Geometry check sheet. Reference: the model listing, model coordinates, mm. Face numbers are marked on the shaded views. Coordinates: 2 decimals unless noted, no trailing zeros. Loops run counter-clockwise (first coordinate to the right, second up) from the corner with the lowest first, then second, coordinate; pieces in that order, holes last. Notation, with made-up numbers: (26.5, 82.25) - (61.5, 82.25) arc R22 cw to (61.5, 102.25) - close; hole circle Ø11 at (87, 64.25). An arc over 180 degrees is marked (long way). One line per item, written item: value.
from build123d import *

# Parameters (mm, degrees)
SKETCH_1_R          = 12.5
SKETCH_1_R_2        = 4
SKETCH_1_R_3        = 1.2
EXTRUDE_1_DEPTH     = 1.2
SKETCH_3_R          = 6
CUT_EXTRUDE_2_DEPTH = 0.3


with BuildPart() as part:
    # 草图1 → 凸台-拉伸1 (new body)
    with BuildSketch(Plane.XY):
        Circle(SKETCH_1_R)
        Circle(SKETCH_1_R_2, mode=Mode.SUBTRACT)
        with Locations((0, -7.5)):
            Circle(SKETCH_1_R_3, mode=Mode.SUBTRACT)
        with Locations((-6.495190528, 3.75)):
            Circle(SKETCH_1_R_3, mode=Mode.SUBTRACT)
        with Locations((6.495190528, 3.75)):
            Circle(SKETCH_1_R_3, mode=Mode.SUBTRACT)
    extrude(amount=EXTRUDE_1_DEPTH)

    # 草图3 → 切除-拉伸2 (cut)
    with BuildSketch(Plane.XY.offset(1.2)):
        Circle(SKETCH_3_R)
    extrude(amount=-CUT_EXTRUDE_2_DEPTH, mode=Mode.SUBTRACT)


solid = part.part
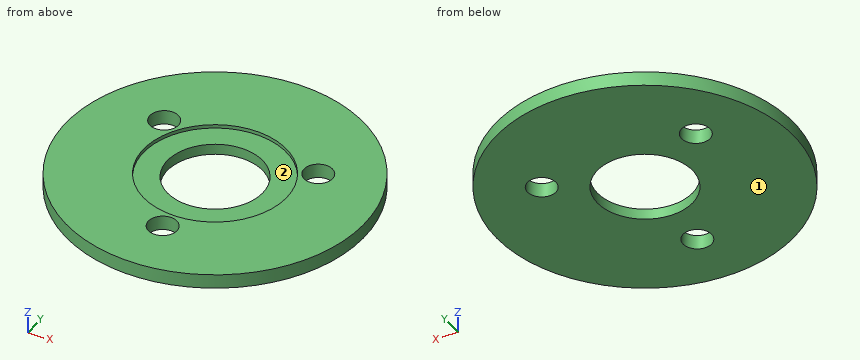
(1) Cross-section at A-A on y = 0. Record the cut outline in (x, z), and give its area (3 significant figures).
Reply:
outline: (-12.5, 0) - (-4, 0) - (-4, 0.9) - (-6, 0.9) - (-6, 1.2) - (-12.5, 1.2) - close; (4, 0) - (12.5, 0) - (12.5, 1.2) - (6, 1.2) - (6, 0.9) - (4, 0.9) - close
area: 19.2 mm2
(2) Cross-section at B-B on x = 0. Record the cut outline in (y, z).
Reply:
outline: (-12.5, 0) - (-8.7, 0) - (-8.7, 1.2) - (-12.5, 1.2) - close; (-6.3, 0) - (-4, 0) - (-4, 0.9) - (-6, 0.9) - (-6, 1.2) - (-6.3, 1.2) - close; (4, 0) - (12.5, 0) - (12.5, 1.2) - (6, 1.2) - (6, 0.9) - (4, 0.9) - close
(3) Cross-section at C-C on z = 0.65. Record the cut outline in (x, y), and give its area (3 significant figures).
Reply:
outline: circle Ø25 at (0, 0); hole circle Ø2.4 at (-6.5, 3.75); hole circle Ø8 at (0, 0); hole circle Ø2.4 at (0, -7.5); hole circle Ø2.4 at (6.5, 3.75)
area: 427 mm2
(4) Cross-section at D-D on x = -2.5. Record the cut outline in (y, z), and give its area (3 significant figures).
Reply:
outline: (-12.25, 0) - (-3.12, 0) - (-3.12, 0.9) - (-5.45, 0.9) - (-5.45, 1.2) - (-12.25, 1.2) - close; (3.12, 0) - (12.25, 0) - (12.25, 1.2) - (5.45, 1.2) - (5.45, 0.9) - (3.12, 0.9) - close
area: 20.5 mm2
(5) Release check for a two-part mould opening along Y. For the marked faces 1 and 2 record: pulls with the +Y half, pulls with the -Y half, needs draft (parallel to the pull), parting line crosses it, or undercut.
Reply:
face 1: needs draft
face 2: undercut
(6) Go/stop test with a flat-tipped pin: pin 1 Ø10.5 at (x, y) = (0, 0) entering from +Z. Record where the tip stops, or that it passes through.
Reply:
pin 1: z = 0.9
(7) Material ranges on probe 1 along Y at (x, z) = (0, 1); probe 2 along X at (y, z) = (-4.5, 1); probe 3 along X at (y, z) = (-3, 0.5), recorded low to high. Write a range as from..to.
Reply:
probe 1: -12.5..-8.7, -6.3..-6, 6..12.5
probe 2: -11.66..-3.97, 3.97..11.66
probe 3: -12.13..-2.65, 2.65..12.13
